Can you work these out from the model? Positions are in its coordinate system, mm. A direction names the side the tool comes from. Give positions to 0.01 mm unless a question says otherwise; leave off trailing zeros. Order: outer loops, then holes, each group sorted by start corner. A loop starts at its lowest first (then second) coordinate and runs counter-clockwise, first axis right, second up. Notation, with made-up numbers: (14, 7) -> (61, 7) arc R24 cw to (61, 19) -> close; hole circle Ø9 at (86.25, 60.25). An arc over 180 degrees is marked (long way). Answer as a JSON object with one key per item and string values.
```python
from build123d import *

# Parameters (mm, degrees)
F0_R     = 132.461
F0_R_2   = 124.1425
F0_R_3   = 9.525
F0_R_4   = 60.1091
F0_R_5   = 5.2832
F1_DEPTH = 8.5852
F2_R     = 9.525
F2_R_2   = 5.2832
F3_DEPTH = 3.048
F5_DEPTH = 8.5862


with BuildPart() as f1:
    # F0 (on Top) → F1 (new body)
    with BuildSketch(Plane.XY):
        Circle(F0_R)
        Circle(F0_R_2, mode=Mode.SUBTRACT)
        Circle(F0_R_2)
        with Locations((-41.1389134724, -56.6228567312)):
            Circle(F0_R_3, mode=Mode.SUBTRACT)
        with Locations((41.1389134724, -56.6228567312)):
            Circle(F0_R_3, mode=Mode.SUBTRACT)
        with Locations((-66.5641602585, 21.6280067312)):
            Circle(F0_R_3, mode=Mode.SUBTRACT)
        Circle(F0_R_4, mode=Mode.SUBTRACT)
        with Locations((66.5641602585, 21.6280067312)):
            Circle(F0_R_3, mode=Mode.SUBTRACT)
        with Locations((0, 69.9897)):
            Circle(F0_R_3, mode=Mode.SUBTRACT)
        with Locations((0, 69.9897)):
            Circle(F0_R_3)
        with Locations((0, 69.9897)):
            Circle(F0_R_5, mode=Mode.SUBTRACT)
        with Locations((66.5641602585, 21.6280067312)):
            Circle(F0_R_3)
        with Locations((66.5641602585, 21.6280067312)):
            Circle(F0_R_5, mode=Mode.SUBTRACT)
        with Locations((41.1389134724, -56.6228567312)):
            Circle(F0_R_3)
        with Locations((41.1389134724, -56.6228567312)):
            Circle(F0_R_5, mode=Mode.SUBTRACT)
        with Locations((-41.1389134724, -56.6228567312)):
            Circle(F0_R_3)
        with Locations((-41.1389134724, -56.6228567312)):
            Circle(F0_R_5, mode=Mode.SUBTRACT)
        with Locations((-66.5641602585, 21.6280067312)):
            Circle(F0_R_3)
        with Locations((-66.5641602585, 21.6280067312)):
            Circle(F0_R_5, mode=Mode.SUBTRACT)
    extrude(amount=F1_DEPTH)

    # F2 (on face) → F3 (cut)
    with BuildSketch(Plane.XY.offset(8.5852)):
        with Locations((-66.5641602585, 21.6280067312)):
            Circle(F2_R)
        with Locations((-66.5641602585, 21.6280067312)):
            Circle(F2_R_2, mode=Mode.SUBTRACT)
        with Locations((0, 69.9897)):
            Circle(F2_R)
        with Locations((0, 69.9897)):
            Circle(F2_R_2, mode=Mode.SUBTRACT)
        with Locations((66.5641602585, 21.6280067312)):
            Circle(F2_R)
        with Locations((66.5641602585, 21.6280067312)):
            Circle(F2_R_2, mode=Mode.SUBTRACT)
        with Locations((41.1389134724, -56.6228567312)):
            Circle(F2_R)
        with Locations((41.1389134724, -56.6228567312)):
            Circle(F2_R_2, mode=Mode.SUBTRACT)
        with Locations((-41.1389134724, -56.6228567312)):
            Circle(F2_R)
        with Locations((-41.1389134724, -56.6228567312)):
            Circle(F2_R_2, mode=Mode.SUBTRACT)
    extrude(amount=-F3_DEPTH, mode=Mode.SUBTRACT)

    # F4 (on face) → F5 (cut, through all)
    with BuildSketch(Plane.XY.offset(8.5852)):
        with BuildLine():
            ThreePointArc((-51.6774888153, 51.2893964924), (-41.8372341216, 59.5886808368), (-30.6891923649, 66.0252869346))
            ThreePointArc((-30.6891923649, 66.0252869346), (-27.7167624168, 68.8833558466), (-27.1264884478, 72.9644677469))
            Line((-27.1264884478, 72.9644677469), (-32.0624553632, 99.0450873522))
            ThreePointArc((-32.0624553632, 99.0450873522), (-35.2275731763, 103.4205413877), (-40.6159999389, 103.7775089083))
            ThreePointArc((-40.6159999389, 103.7775089083), (-53.4701008219, 97.7771912275), (-65.45782702, 90.1925922017))
            ThreePointArc((-65.45782702, 90.1925922017), (-67.6298177949, 87.3968028542), (-67.9672788915, 83.8725863441))
            Line((-67.9672788915, 83.8725863441), (-62.4237511818, 54.5817422306))
            ThreePointArc((-62.4237511818, 54.5817422306), (-58.0446252801, 49.6911222717), (-51.6774888153, 51.2893964924))
        make_face()
        with BuildLine():
            ThreePointArc((53.3102973951, 49.5900920997), (56.9470138263, 47.6463350933), (61.0107865806, 48.3460841217))
            Line((61.0107865806, 48.3460841217), (84.2896321448, 61.0998223028))
            ThreePointArc((84.2896321448, 61.0998223028), (87.4728610235, 65.4621178788), (86.1472418675, 70.6971252943))
            ThreePointArc((86.1472418675, 70.6971252943), (76.468465017, 81.0679015652), (65.550671571, 90.125136687))
            ThreePointArc((65.550671571, 90.125136687), (62.2205358328, 91.3268762457), (58.7645255422, 90.5587780272))
            Line((58.7645255422, 90.5587780272), (32.6203216513, 76.2352012649))
            ThreePointArc((32.6203216513, 76.2352012649), (29.3222899949, 70.55912036), (32.8098924804, 64.997507631))
            ThreePointArc((32.8098924804, 64.997507631), (43.743786866, 58.203489186), (53.3102973951, 49.5900920997))
        make_face()
        with BuildLine():
            ThreePointArc((63.6367681054, -35.3769245118), (62.9119525193, -39.4363013195), (64.8332282349, -43.0849445367))
            Line((64.8332282349, -43.0849445367), (84.1563129279, -61.2833204626))
            ThreePointArc((84.1563129279, -61.2833204626), (89.288774382, -62.9627275631), (93.8579234501, -60.0842825695))
            ThreePointArc((93.8579234501, -60.0842825695), (100.73021127, -47.6744726636), (105.9703700363, -34.4921944885))
            ThreePointArc((105.9703700363, -34.4921944885), (106.0842237378, -30.953689248), (104.2857530094, -27.9041835437))
            Line((104.2857530094, -27.9041835437), (82.5842186863, -7.4657967097))
            ThreePointArc((82.5842186863, -7.4657967097), (76.1667971249, -6.0831876729), (71.9551175354, -11.1187275924))
            ThreePointArc((71.9551175354, -11.1187275924), (68.8723812014, -23.616946256), (63.6367681054, -35.3769245118))
        make_face()
        with BuildLine():
            ThreePointArc((-72.2772613638, -8.7842206572), (-74.076915058, -5.074079921), (-77.7758784367, -3.2515630831))
            Line((-77.7758784367, -3.2515630831), (-104.105319322, 0.1134080996))
            ThreePointArc((-104.105319322, 0.1134080996), (-109.2446985876, -1.5447081663), (-111.2493103168, -6.5590975212))
            ThreePointArc((-111.2493103168, -6.5590975212), (-109.5148047069, -20.6382740621), (-106.0058334991, -34.3830491728))
            ThreePointArc((-106.0058334991, -34.3830491728), (-104.018061883, -37.3126815737), (-100.77061402, -38.7226689421))
            Line((-100.77061402, -38.7226689421), (-71.2003215869, -42.5018294012))
            ThreePointArc((-71.2003215869, -42.5018294012), (-65.1958412822, -39.848317857), (-64.7483370215, -33.2989173362))
            ThreePointArc((-64.7483370215, -33.2989173362), (-69.6006195485, -21.3756590841), (-72.2772613638, -8.7842206572))
        make_face()
        with BuildLine():
            ThreePointArc((-13.9806117717, -71.4542338654), (-18.0652888708, -72.0193096994), (-20.941647931, -74.9740442488))
            Line((-20.941647931, -74.9740442488), (-32.2781703875, -98.9749972921))
            ThreePointArc((-32.2781703875, -98.9749972921), (-32.2893636416, -104.3752235372), (-28.1398550618, -107.8312541119))
            ThreePointArc((-28.1398550618, -107.8312541119), (-14.2137707582, -110.532346067), (-0.0573810882, -111.4424852274))
            ThreePointArc((-0.0573810882, -111.4424852274), (3.3431201074, -110.4573082782), (5.68761436, -107.8045118855))
            Line((5.68761436, -107.8045118855), (18.4195324312, -80.8493173845))
            ThreePointArc((18.4195324312, -80.8493173845), (17.7513794425, -74.3187371018), (11.660815821, -71.8692591947))
            ThreePointArc((11.660815821, -71.8692591947), (-1.1783143974, -72.7995646827), (-13.9806117717, -71.4542338654))
        make_face()
    extrude(amount=-F5_DEPTH, mode=Mode.SUBTRACT)


solid = f1.part
```
1. If we section it at B-B on y = 36: Please give me the cut outline in (x, z), then the cut area to 3 significant figures.
Worked answers:
{"outline": "(-127.48, 0) -> (-48.14, 0) -> (-48.14, 8.59) -> (-127.48, 8.59) -> close; (48.14, 0) -> (127.48, 0) -> (127.48, 8.59) -> (48.14, 8.59) -> close", "area": "1,360 mm²"}
2. If we section it at D-D on x = 109.5: Please give me the cut outline in (y, z), then the cut area to 3 significant figures.
Worked answers:
{"outline": "(-74.54, 0) -> (74.54, 0) -> (74.54, 8.59) -> (-74.54, 8.59) -> close", "area": "1,280 mm²"}
3. For faces 1 (the face through (71, 18, 5.537)), 2 (the face through (106.096, -31.002, 4.353)), which set-ups out of +Z, -Z, +X, -X, +Y, -Y let a thin tool reach every point of the face, with its end or its side?
Worked answers:
{"face 1": "+Z", "face 2": "+Z, -Z"}
4. Please list where these lines run through material, in increasing order: L1, parallel to Y at x = 1.5, z = 2.75; L2, parallel to Y at x = -55, z = 0.5; L3, parallel to X at y = 82.5, z = 0.5.
Worked answers:
{"L1": "-132.45 to -111.25, -72.79 to -60.09, 60.09 to 64.92, 75.06 to 132.45", "L2": "-120.5 to -24.25, 24.25 to 49.52, 96.92 to 120.5", "L3": "-103.63 to -67.71, -28.93 to 44.06, 74.92 to 103.63"}
5. Will these pins go through, and if not, where does the flat tip stop? pin 1 Ø12 at (x, y) = (41.14, -56.62) entering from +Z; pin 2 Ø2 at (y, z) = (-42.5, 6.5) entering from +X; pin 3 Ø3 at (y, z) = (-24, 1) entering from +X; pin 4 Ø6.5 at (x, y) = (66.56, 21.63) entering from +Z.
Worked answers:
{"pin 1": "z = 5.54", "pin 2": "x = 125.79", "pin 3": "x = 130.54", "pin 4": "through"}
6. If we section it at A-A on x = 23: Please give me the cut outline in (y, z), then the cut area to 3 significant figures.
Worked answers:
{"outline": "(-130.45, 0) -> (-55.53, 0) -> (-55.53, 8.59) -> (-130.45, 8.59) -> close; (55.53, 0) -> (130.45, 0) -> (130.45, 8.59) -> (55.53, 8.59) -> close", "area": "1,290 mm²"}
7. If we section it at C-C on z = 2: Count the separate pieces of the cut face and the enclosed holes in it, then the cut area to 3 significant figures.
Worked answers:
{"separate pieces": "1", "enclosed holes": "11", "area": "35,600 mm²"}
